Check sheet for the modelled part. Datum: model origin and axes. Units: mm. Face numbers are marked on the shaded views. A direction names the side the tool comes from. Coordinates: 2 decimals unless noted, no trailing zeros. One line per item, written item: value. Start each with the question number.
1) Scan lines: line 1 along Z through (x, y) = (18.5, -34); line 2 along Y through (x, z) = (9, 4.5); line 3 along Z through (x, y) = (23, -17.5). Record each from-to range of solid material in increasing order. Write a range as [from, to].
2) Gauge pin test, flat ends, axial feed: P1, Ø1.1, axis at y = -8.5, z = 5, coming from the -X side; P2, Ø1.1, axis at x = 10, z = 4, coming from the +Y side. Record the tip position at first contact, or that the pin passes through.
3) Draft check along X on the marked faces 1, 2, 3 and 4. Enter one of: +X half, -X half, draft (parallel to the pull), parting line (faces both ways), or undercut.
4) Set-up check for the marked faces 5 and 6: record each of +Z, -Z, +X, -X, +Y, -Y from which the full face is reachable in a straight line by a thin tool's end or side.
```python
from build123d import *

# Parameters (mm, degrees)
F0_W        = 30
F0_H        = 40
F1_DEPTH    = 8
F2_R        = 12
F3_R        = 5
F5_DEPTH    = 25
F4_W        = 26.9999996879
F4_H        = 0.8
F4_W_2      = 3.0000003121
F6_DEPTH    = 1
F7_T1_DEPTH = 8
F8_R        = 3
F9_R        = 2
F10_R       = 0.5
F11_R       = 1
F12_R       = 7.0500114294
F13_DEPTH   = 0.2


# Not quite as in the source:
# - a fillet or chamfer that OpenCascade refuses, or shapes differently, is made with other operations: its cross-section is extruded or revolved along the edge and cut away or added


with BuildPart() as f1:
    # F0 (on Top) → F1 (new body)
    with BuildSketch(Plane.XY):
        with Locations((15, -20)):
            Rectangle(F0_W, F0_H)
    extrude(amount=F1_DEPTH)

    # F2
    f2_edges = [f1.edges().sort_by_distance(p)[0] for p in [
        (0, 0, 4),
    ]]
    fillet(f2_edges, radius=F2_R)

    # F3
    f3_edges = [f1.edges().sort_by_distance(p)[0] for p in [
        (30, 0, 4),
        (30, -40, 4),
        (0, -40, 4),
    ]]
    fillet(f3_edges, radius=F3_R)

    # F4 (on face) → F5 (cut)
    with BuildSketch(Plane.XY.offset(8)):
        with BuildLine():
            Line((3.0000003121, -12), (3.0000003121, -13.0000003121))
            Line((3.0000003121, -13.0000003121), (13.0000003121, -13.0000003121))
            Line((13.0000003121, -13.0000003121), (13.0000003121, -3.0000003121))
            Line((13.0000003121, -3.0000003121), (12, -3.0000003121))
            ThreePointArc((12, -3.0000003121), (5.63603919, -5.63603919), (3.0000003121, -12))
        make_face()
    extrude(amount=-F5_DEPTH, mode=Mode.SUBTRACT)

    # F4 (on face) → F6 (cut)
    with BuildSketch(Plane.XY.offset(8)):
        with Locations((16.500000156, -17.6)):
            Rectangle(F4_W, F4_H)
        with Locations((1.500000156, -17.6)):
            Rectangle(F4_W_2, F4_H)
    extrude(amount=-F6_DEPTH, mode=Mode.SUBTRACT)

    # F7: fillet of radius 10 on 2 edges, made by hand

    # F7_s2 → F7_t1 (join)
    with BuildSketch(Plane.XY):
        with BuildLine():
            ThreePointArc((13.0000003121, -7.3588999), (12.7467945768, -5.1228315736), (12, -3.0000003121))
            Line((12, -3.0000003121), (13.0000003121, -3.0000003121))
            Line((13.0000003121, -3.0000003121), (13.0000003121, -7.3588999))
        make_face()
        with BuildLine():
            ThreePointArc((3.0000003121, -12), (5.1228315736, -12.7467945768), (7.3588999, -13.0000003121))
            Line((7.3588999, -13.0000003121), (3.0000003121, -13.0000003121))
            Line((3.0000003121, -13.0000003121), (3.0000003121, -12))
        make_face()
    extrude(amount=F7_T1_DEPTH)

    # F8
    f8_edges = [f1.edges().sort_by_distance(p)[0] for p in [
        (12, -3, 4),
        (3, -12, 4),
    ]]
    fillet(f8_edges, radius=F8_R)

    # F9
    f9_edges = [f1.edges().sort_by_distance(p)[0] for p in [
        (13, -13, 4),
    ]]
    fillet(f9_edges, radius=F9_R)

    # F10
    f10_edges = [f1.edges().sort_by_distance(p)[0] for p in [
        (30, -11.1, 8),
        (30, -26.5, 8),
        (30, -20, 0),
        (18.5, 0, 0),
        (3.514719, -3.514719, 0),
        (0, -23.5, 0),
        (1.464466, -38.535534, 0),
        (15, -40, 0),
        (28.535534, -38.535534, 0),
        (28.535534, -1.464466, 0),
        (18.5, 0, 8),
        (3.514719, -3.514719, 8),
        (0, -26.5, 8),
        (0, -14.6, 8),
        (1.464466, -38.535534, 8),
        (15, -40, 8),
        (28.535534, -38.535534, 8),
        (28.535534, -1.464466, 8),
    ]]
    fillet(f10_edges, radius=F10_R)

    # F11
    f11_edges = [f1.edges().sort_by_distance(p)[0] for p in [
        (5.636039, -5.636039, 8),
        (11.467525, -3.792736, 0),
        (9.17945, -13, 0),
        (12.414214, -12.414214, 0),
        (6.649711, -12.974821, 0),
        (13, -9.17945, 0),
        (3.792736, -11.467525, 0),
        (12.974821, -6.649711, 0),
        (5.636039, -5.636039, 0),
        (9.17945, -13, 8),
        (12.414214, -12.414214, 8),
        (6.649711, -12.974821, 8),
        (13, -9.17945, 8),
        (3.792736, -11.467525, 8),
        (12.974821, -6.649711, 8),
        (11.467525, -3.792736, 8),
    ]]
    fillet(f11_edges, radius=F11_R)

    # F12 (on face) → F13 (cut)
    with BuildSketch(Plane.XY.offset(8)):
        with Locations((15.0601761416, -28.3769778907)):
            Circle(F12_R)
    extrude(amount=-F13_DEPTH, mode=Mode.SUBTRACT)


solid = f1.part
```
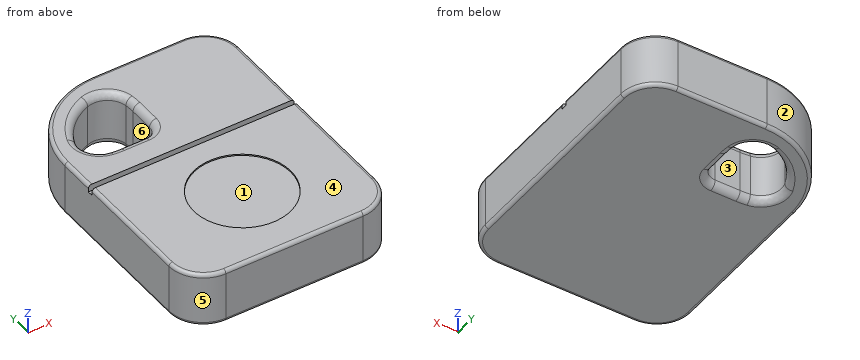
Answers:
1. line 1: z = [0, 7.8]
1. line 2: y = [-40, -13], [-3.52, -0.38]
1. line 3: z = [0, 7]
2. P1: stops at x = 0.37
2. P2: stops at y = -0.09
3. face 1: undercut
3. face 2: -X half
3. face 3: undercut
3. face 4: draft
4. face 5: +Z, -Z, -X, -Y
4. face 6: +Z, -Z
